from build123d import *

# Parameters (mm, degrees)
CYLINDER003_R     = 11
CYLINDER003_DEPTH = 15
CYLINDER001_R     = 1.5
CYLINDER001_DEPTH = 25
CYLINDER_R        = 4
CYLINDER_DEPTH    = 25
CYLINDER002_R     = 1.5
CYLINDER002_DEPTH = 25
BOX_W             = 50
BOX_H             = 65
BOX_DEPTH         = 18


with BuildPart() as cilindro003:
    # Cylinder003 → Cylinder003 (new body)
    with BuildSketch(Plane(origin=(50, 7, 10), x_dir=(1, 0, 0), z_dir=(0, 0, 1))):
        Circle(CYLINDER003_R)
    extrude(amount=CYLINDER003_DEPTH)


with BuildPart() as cilindro001:
    # Cylinder001 → Cylinder001 (new body)
    with BuildSketch(Plane(origin=(20, 52, 0), x_dir=(1, 0, 0), z_dir=(0, 0, 1))):
        Circle(CYLINDER001_R)
    extrude(amount=CYLINDER001_DEPTH)


with BuildPart() as cilindro:
    # Cylinder → Cylinder (new body)
    with BuildSketch(Plane(origin=(18, 7, 8), x_dir=(1, 0, 0), z_dir=(0, 0, 1))):
        Circle(CYLINDER_R)
    extrude(amount=CYLINDER_DEPTH)


with BuildPart() as fusion:
    # Cylinder002 → Cylinder002 (new body)
    with BuildSketch(Plane(origin=(20, 60, 0), x_dir=(1, 0, 0), z_dir=(0, 0, 1))):
        Circle(CYLINDER002_R)
    extrude(amount=CYLINDER002_DEPTH)

    # Fusion: union Cilindro001, Cilindro
    add(cilindro001.part)
    add(cilindro.part)


with BuildPart() as izquierda:
    # Box → Box (new body)
    with BuildSketch(Plane.XY):
        with Locations((25, 32.5)):
            Rectangle(BOX_W, BOX_H)
    extrude(amount=BOX_DEPTH)

    # Cut: cut Fusion
    add(fusion.part, mode=Mode.SUBTRACT)


with BuildPart() as z_abajo:
    # mirror: instance of Izquierda
    add(izquierda.part.mirror(Plane(origin=(50, 0, 0), x_dir=(0, -1, 0), z_dir=(1, 0, 0))))

    # Fusion001: union Izquierda
    add(izquierda.part)

    # Cut001: cut Cilindro003
    add(cilindro003.part, mode=Mode.SUBTRACT)


solid = z_abajo.part
For this review, take the finished solid that the model builds, in its own axes (mm). A direction names the side the tool comes from. Coordinates: 2 decimals unless noted, no trailing zeros. Loops run counter-clockwise (first coordinate to the right, second up) from the corner with the lowest first, then second, coordinate; pieces in that order, holes last. Notation, with made-up numbers: (71, -18) - (110, -18) arc R34 cw to (110, 15) - close; hole circle Ø8 at (24.5, 4.25). An arc over 180 degrees is marked (long way). Return JSON: item names as keys, results as strings.
Item 1: Take a section at A-A (y = 7). Give the boundary of the cut face in (x, z).
Determined:
{"outline": "(0, 0) - (100, 0) - (100, 18) - (86, 18) - (86, 8) - (78, 8) - (78, 18) - (61, 18) - (61, 10) - (39, 10) - (39, 18) - (22, 18) - (22, 8) - (14, 8) - (14, 18) - (0, 18) - close"}
Item 2: Mouldability with a two-part tool opening along X and no side actions: class faces 3 (the flat face through (49, 33, 0)), 4 (the flat face through (82, 7, 8)), 5 (the flat face through (0, 32, 9)) as pulls with the +X half, pulls with the -X half, needs draft (parallel to the pull), parting line crosses it, or undercut.
Determined:
{"face 3": "needs draft", "face 4": "undercut", "face 5": "pulls with the -X half"}
Item 3: Insertion check: pin 1 (9 mm diameter, centred on x = 45.5, y = 8.5, fed in from +Z); pin 2 (4 mm diameter, centred on x = 81.5, y = 6, fed in from +Z); pin 3 (1.8 mm diameter, centred on x = 20, y = 60, fed in from -Z). Each pin has a flat end and moves straight along its axis. Give the tip position at first contact, or say it passes through.
Determined:
{"pin 1": "stops at z = 10", "pin 2": "stops at z = 8", "pin 3": "passes through"}
Item 4: Take a section at B-B (x = 80). Give the boundary of the cut face in (y, z), then the cut area to 3 significant figures.
Determined:
{"outline": "(0, 0) - (50.5, 0) - (50.5, 18) - (10.46, 18) - (10.46, 8) - (3.54, 8) - (3.54, 18) - (0, 18) - close; (53.5, 0) - (58.5, 0) - (58.5, 18) - (53.5, 18) - close; (61.5, 0) - (65, 0) - (65, 18) - (61.5, 18) - close", "area": "993 mm2"}
Item 5: For faces 1 (the cylindrical face through (18.89, 61.01, 8.87)), 2 (the cylindrical face through (86, 7, 13)), list the 3-axis set-ups (+Z, -Z, +X, -X, +Y, -Y) from which the entire face can be reached by the end or side of a thin tool; tool diameter is ignored.
Determined:
{"face 1": "+Z, -Z", "face 2": "+Z"}
Item 6: Take a section at C-C (y = 52). Give the boundary of the cut face in (x, z).
Determined:
{"outline": "(0, 0) - (18.5, 0) - (18.5, 18) - (0, 18) - close; (21.5, 0) - (78.5, 0) - (78.5, 18) - (21.5, 18) - close; (81.5, 0) - (100, 0) - (100, 18) - (81.5, 18) - close"}
Item 7: Take a section at D-D (z = 15.5). Give the boundary of the cut face in (x, y), then the cut area to 3 significant figures.
Determined:
{"outline": "(0, 0) - (41.51, 0) arc R11 cw (long way) to (58.49, 0) - (100, 0) - (100, 65) - (0, 65) - close; hole circle Ø8 at (18, 7); hole circle Ø3 at (20, 52); hole circle Ø3 at (20, 60); hole circle Ø8 at (82, 7); hole circle Ø3 at (80, 52); hole circle Ø3 at (80, 60)", "area": "6,040 mm2"}
Item 8: For line 1 (Y direction, x = 20, z = 14); line 2 (Y direction, x = 82, z = 13); line 3 (Y direction, x = 19.5, z = 17.25), list the stretches that pass through material, from the lowest coordinate up.
Determined:
{"line 1": "y = 0 to 3.54, 10.46 to 50.5, 53.5 to 58.5, 61.5 to 65", "line 2": "y = 0 to 3, 11 to 65", "line 3": "y = 0 to 3.29, 10.71 to 50.59, 53.41 to 58.59, 61.41 to 65"}
